Geometry check sheet. Reference: the model listing, model coordinates, mm. Face numbers are marked on the shaded views. Round coordinates to 2 decimals unless told otherwise and drop trailing zeros. Loops run counter-clockwise (first coordinate to the right, second up) from the corner with the lowest first, then second, coordinate; pieces in that order, holes last. Notation, with made-up numbers: M 33.25,21.25 L 91.25,21.25 A23 cw 91.25,48.25 Z; hole C 33,59 d7. An arc over 180 degrees is marked long. Answer in a Markdown table with one row per item. Add a question column.
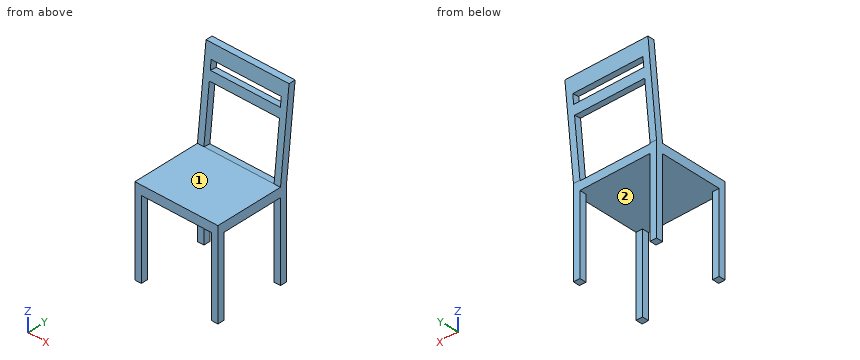
```python
from build123d import *

# Parameters (mm, degrees)
F0_W     = 450
F0_H     = 450
F1_DEPTH = 950
F2_W     = 50
F2_H     = 50
F2_W_2   = 329.8066283627
F2_H_2   = 425
F3_DEPTH = 450.001
F4_W     = 380
F4_H     = 425
F5_DEPTH = 450.001
F6_W     = 380
F6_H     = 302.6243293636
F6_H_2   = 50
F7_DEPTH = 134.4515452921


with BuildPart() as f1:
    # F0 (on Top) → F1 (new body)
    with BuildSketch(Plane.XY):
        Rectangle(F0_W, F0_H)
    extrude(amount=F1_DEPTH)

    # F2 (on face) → F3 (cut, through all)
    with BuildSketch(Plane.YZ.offset(225)):
        with Locations((200, 450)):
            Rectangle(F2_W, F2_H)
        Polygon((-225, 950), (-225, 475), (139.8066283627, 475), (189.8066283627, 950), align=None)
        Polygon((225, 950), (175, 475), (225, 475), align=None)
        with Locations((-25.0966858187, 212.5)):
            Rectangle(F2_W_2, F2_H_2)
        with Locations((200, 212.5)):
            Rectangle(F2_W, F2_H_2)
    extrude(amount=-F3_DEPTH, mode=Mode.SUBTRACT)

    # F4 (on face) → F5 (cut, through all)
    with BuildSketch(Plane.XZ.offset(225)):
        with Locations((0, 212.5)):
            Rectangle(F4_W, F4_H)
    extrude(amount=-F5_DEPTH, mode=Mode.SUBTRACT)

    # F6 (on face) → F7 (cut, through all)
    with BuildSketch(Plane(origin=(0, 88.8224461341, -9.349731172), x_dir=(1, 0, 0), z_dir=(0, -0.9945054529, 0.1046847845))):
        with Locations((0, 638.3378815838)):
            Rectangle(F6_W, F6_H)
        with Locations((0, 864.6500462656)):
            Rectangle(F6_W, F6_H_2)
    extrude(amount=-F7_DEPTH, mode=Mode.SUBTRACT)


solid = f1.part
```
1) Cross-section at A-A, the plane z = 288.5. Record the boundary of the cut face in (x, y).
2) Draft check along Y on the marked faces 1 and 2. Enter one of: +Y half, -Y half, draft (parallel to the pull), parting line (faces both ways), or undercut.
3) Cross-section at B-B, the plane x = -153. Record the boundary of the cut face in (y, z), plus the area to 3 significant figures.
4) Go/stop test with flat-tipped pins: pin 1 (2 mm diameter, centred on x = -136.5, y = -47.5, fed in from +Z); pin 2 (6 mm diameter, centred on x = -33.5, y = 130.5, fed in from -Z); pin 3 (10.5 mm diameter, centred on x = -203, z = 235.5, fed in from +Y). Record where each tip stops, or that it passes through.
5) Cross-section at C-C, the plane z = 580. Record the boundary of the cut face in (x, y).
6) Cross-section at D-D, the plane y = 160.5. Record the boundary of the cut face in (x, z), plus the area to 3 significant figures.
7) Thickness scan on L1, parallel to Z at x = 19, y = -64.5; L2, parallel to Y at x = -200.5, z = 871.5. Record the ranges inside material, lowest first. Write a range as [from, to].
Worked answers:
| question | item | result |
|---|---|---|
| 1 | outline | M -225,-225 L -190,-225 L -190,-190 L -225,-190 Z; M -225,139.81 L -190,139.81 L -190,175 L -225,175 Z; M 190,-225 L 225,-225 L 225,-190 L 190,-190 Z; M 190,139.81 L 225,139.81 L 225,175 L 190,175 Z |
| 2 | face 1 | draft |
| 2 | face 2 | undercut |
| 3 | outline | M -225,425 L 175,425 L 175,471.3 L 139.81,475 L -225,475 Z; M 171.49,775.96 L 206.29,772.3 L 211.53,822.02 L 176.72,825.69 Z; M 181.96,875.41 L 216.76,871.75 L 225,950 L 189.81,950 Z |
| 3 | area | 24,400 mm2 |
| 4 | pin 1 | stops at z = 475 |
| 4 | pin 2 | stops at z = 425 |
| 4 | pin 3 | stops at y = 175 |
| 5 | outline | M -225,150.86 L -190,150.86 L -190,186.05 L -225,186.05 Z; M 190,150.86 L 225,150.86 L 225,186.05 L 190,186.05 Z |
| 6 | outline | M -225,0 L -190,0 L -190,425 L 190,425 L 190,0 L 225,0 L 225,671.59 L 190,671.59 L 190,472.82 L -190,472.82 L -190,671.59 L -225,671.59 Z |
| 6 | area | 65,200 mm2 |
| 7 | L1 | z = [425, 475] |
| 7 | L2 | y = [181.54, 216.74] |
